Autodesk Inventor part; units mm, degrees
ref_plane "YZ Plane" through (0, 0, 0) normal (1, 0, 0) x (0, 1, 0)
ref_plane "XZ Plane" through (0, 0, 0) normal (0, 1, 0) x (-1, 0, 0)
ref_plane "XY Plane" through (0, 0, 0) normal (0, 0, 1) x (1, 0, 0)
sketch "Sketch1" plane through (0, 0, 0) normal (1, 0, 0) x (0, 1, 0)
  line L0 (0, 0) -> (52.8273, -113.2885)
  line L1 (0, 0) -> (0, -113.2885)
  circle A0 centre (52.8273, -113.2885) radius 4
  circle A1 centre (0, 0) radius 4
  circle A2 centre (52.8273, -113.2885) radius 8
  circle A3 centre (0, 0) radius 8
  line L2 (60.0777, -109.9075) -> (7.2505, 3.3809)
  circle A4 centre (0, -113.2885) radius 8
  line L3 (-8, 0) -> (-8, -113.2885)
  line L4 (0, -121.2885) -> (52.8273, -121.2885)
  circle A5 centre (0, -113.2885) radius 4
  dimension "d0" = 125
  dimension "d1" = 25
  dimension "d2" = 8
  dimension "d3" = 8
  dimension "d4" = 16
  dimension "d5" = 16
  dimension "d6" = 16
  dimension "d7" = 8
extrude "Extrusion1" add sketch "Sketch1" along normal blind 2.5 contours A1 L1 A3 L0 | L0 A3 L1 A1 | A3 L2 A2 L0 | L0 A2 L4 A4 L1 A3 | L1 A4 L3 A3 | A2 | A4
properties part number "RockerFront"
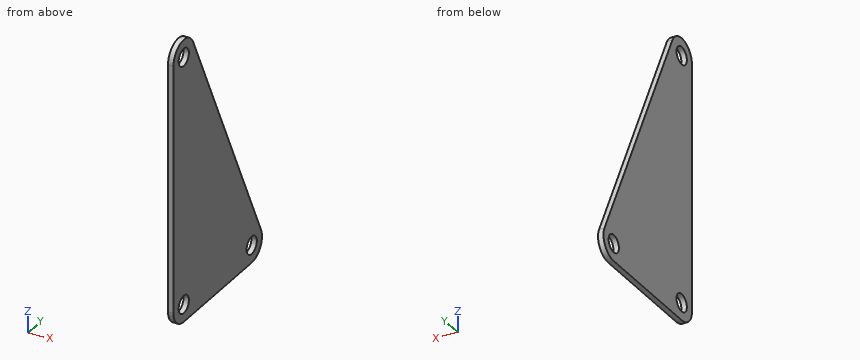
Verification items for the finished model (mm, model axes). Round coordinates to 2 decimals unless told otherwise and drop trailing zeros. Order: outer loops, then holes, each group sorted by start corner. A loop starts at its lowest first (then second) coordinate and runs counter-clockwise, first axis right, second up. Notation, with made-up numbers: (-9, -11.75) -> (24, -11.75) arc R30 cw to (24, 19.25) -> close; hole circle Ø4 at (-15, 31.25). An arc over 180 degrees is marked (long way). Put each result on its own line as item: value. Start each with the question number.
(1) Material ranges on line 1 along Z through (x, y) = (1.15, 0); line 2 along Y through (x, z) = (0.8, -114); line 3 along Z through (x, y) = (1.6, -3.5) (1 decimal), recorded low to high.
(2) Section check B-B (z = -11). Enter the section's corners in (x, y).
(3) Section check C-C (y = 39). Enter the section's corners in (x, z).
(4) Section check A-A (x = 1.5). Enter the section's corners in (y, z), then the cut area to 3 significant figures.
(5) Depth check by flat-ended pin: pin 1 Ø1 at (x, y) = (1.5, 7.5) entering from +Z. Enter the tip coordinate at first touch or a pass-through.
Completed:
1. line 1: z = -121.29 to -117.29, -109.29 to -4, 4 to 8
1. line 2: y = -7.97 to -3.94, 3.94 to 48.89, 56.76 to 60.8
1. line 3: z = -120.5 to -115.2, -111.4 to -1.9, 1.9 to 7.2
2. outline: (0, -8) -> (2.5, -8) -> (2.5, 13.96) -> (0, 13.96) -> close
3. outline: (0, -121.29) -> (2.5, -121.29) -> (2.5, -64.71) -> (0, -64.71) -> close
4. outline: (-8, -113.29) arc R8 ccw to (0, -121.29) -> (52.83, -121.29) arc R8 ccw to (60.08, -109.91) -> (7.25, 3.38) arc R8 ccw to (-8, 0) -> close; hole circle Ø8 at (0, -113.29); hole circle Ø8 at (0, 0); hole circle Ø8 at (52.83, -113.29)
4. area: 5,370 mm2
5. pin 1: stops at z = 3.87
